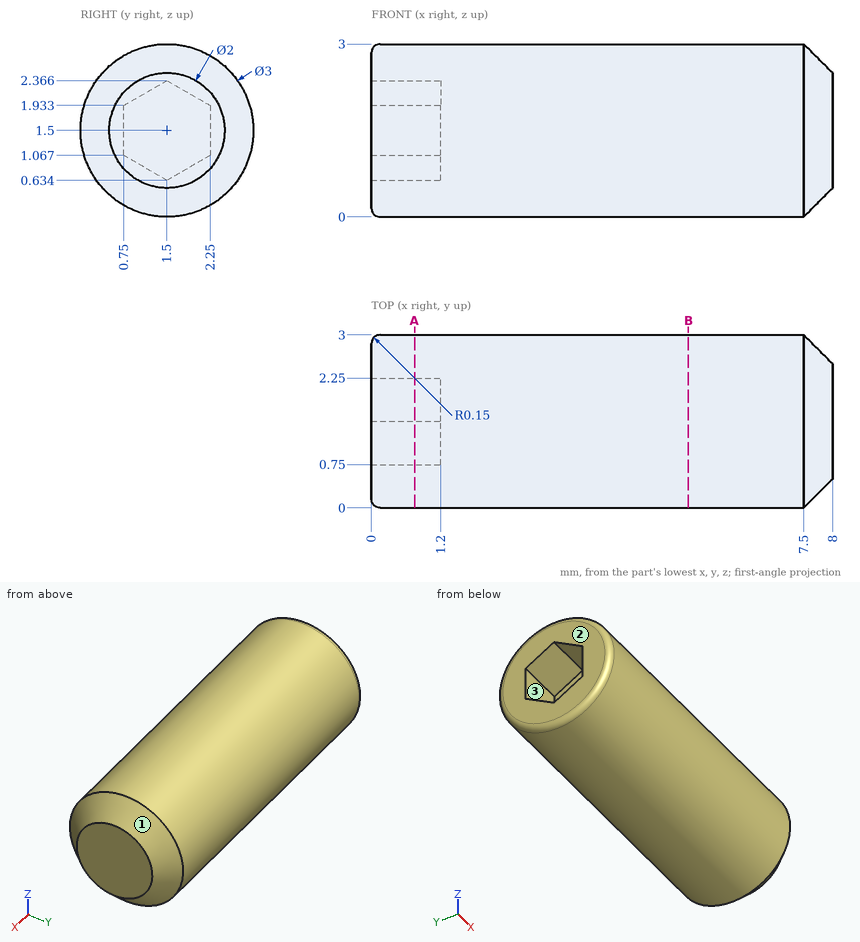
Here's the drawing with two shaded views (mm, measured from the low corner). I have some questions. Coordinates: 2 decimals unless noted, no trailing zeros. Order: outer loops, then holes, each group sorted by start corner. A loop starts at its lowest first (then second) coordinate and runs counter-clockwise, first axis right, second up. Notation, with made-up numbers: (-6.75, -35.5) - (8.25, -35.5) arc R20 ccw to (8.25, -13.5) - close; hole circle Ø3 at (10, 77). An arc over 180 degrees is marked (long way). Answer in a Markdown table with one row per item. Add a question column.
(1) If we section it at A-A, the plane x = 0.75: Please give me the cut outline in (y, z).
(2) If we mould it in two halves opening along Z, with no side actions, what happens to the marked faces 1, 2 and 3? For each: released by +Z, released by -Z, zero draft, split by the parting line, or undercut.
(3) I need wall thicknesses on L1, parallel to Z at x = 2.25, y = 0.2; L2, parallel to X at y = 2, z = 1.1; L3, parallel to Z at x = 3, y = 1.95. Which ranges of each line are inside material? Lowest first, please.
(4) Will these pins go through, and if not, where does the flat tip stop? pin 1 (1.2 mm diameter, centred on y = 1.5, z = 1.5, fed in from -X); pin 2 (1.5 mm diameter, centred on x = 2, z = 0.5, fed in from -Y).
(5) If we section it at B-B, the plane x = 5.5: Please give me the cut outline in (y, z).
Results are:
| question | item | result |
|---|---|---|
| 1 | outline | circle Ø3 at (1.5, 1.5); hole (0.75, 1.07) - (1.5, 0.63) - (2.25, 1.07) - (2.25, 1.93) - (1.5, 2.37) - (0.75, 1.93) - close |
| 2 | face 1 | split by the parting line |
| 2 | face 2 | zero draft |
| 2 | face 3 | undercut |
| 3 | L1 | z = 0.75 to 2.25 |
| 3 | L2 | x = 1.2 to 8 |
| 3 | L3 | z = 0.07 to 2.93 |
| 4 | pin 1 | stops at x = 1.2 |
| 4 | pin 2 | stops at y = 0.02 |
| 5 | outline | circle Ø3 at (1.5, 1.5) |
